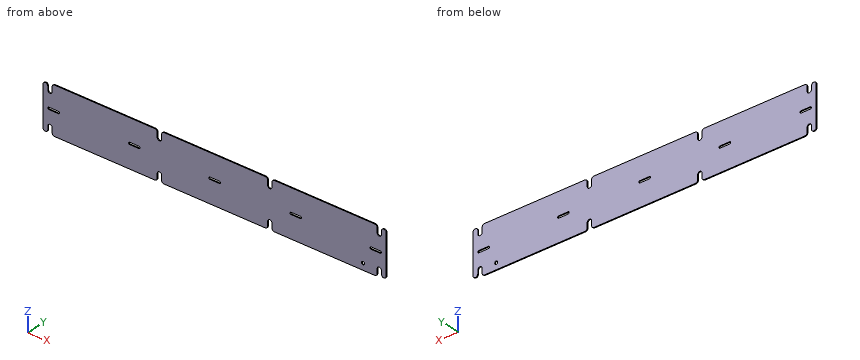
from build123d import *

# Parameters (mm, degrees)
F1_DEPTH = 1
F3_DEPTH = 25
F4_R     = 3.25
F5_DEPTH = 25


with BuildPart() as f1:
    # F0 (on Front) → F1 (new body, symmetric)
    with BuildSketch(Plane.XZ):
        with BuildLine():
            Line((-370, 42.5), (-370, -42.5))
            ThreePointArc((-370, -42.5), (-364.875, -47.501144), (-359.75, -42.5))
            Line((-359.75, -42.5), (-359.75, -35))
            ThreePointArc((-359.75, -35), (-355, -30.25), (-350.25, -35))
            Line((-350.25, -35), (-350.25, -45))
            ThreePointArc((-350.25, -45), (-348.785534, -48.535534), (-345.25, -50))
            Line((-345.25, -50), (-128.75, -50))
            ThreePointArc((-128.75, -50), (-125.214466, -48.535534), (-123.75, -45))
            Line((-123.75, -45), (-123.75, -35))
            ThreePointArc((-123.75, -35), (-119, -30.25), (-114.25, -35))
            Line((-114.25, -35), (-114.25, -45))
            ThreePointArc((-114.25, -45), (-112.785534, -48.535534), (-109.25, -50))
            Line((-109.25, -50), (109.25, -50))
            ThreePointArc((109.25, -50), (112.785534, -48.535534), (114.25, -45))
            Line((114.25, -45), (114.25, -35))
            ThreePointArc((114.25, -35), (119, -30.25), (123.75, -35))
            Line((123.75, -35), (123.75, -45))
            ThreePointArc((123.75, -45), (125.214466, -48.535534), (128.75, -50))
            Line((128.75, -50), (345.25, -50))
            ThreePointArc((345.25, -50), (348.785534, -48.535534), (350.25, -45))
            Line((350.25, -45), (350.25, -35))
            ThreePointArc((350.25, -35), (355, -30.25), (359.75, -35))
            Line((359.75, -35), (359.75, -42.5))
            ThreePointArc((359.75, -42.5), (364.875, -47.501144), (370, -42.5))
            Line((370, -42.5), (370, 42.5))
            ThreePointArc((370, 42.5), (364.875, 47.501144), (359.75, 42.5))
            Line((359.75, 42.5), (359.75, 35))
            ThreePointArc((359.75, 35), (355, 30.25), (350.25, 35))
            Line((350.25, 35), (350.25, 45))
            ThreePointArc((350.25, 45), (348.785534, 48.535534), (345.25, 50))
            Line((345.25, 50), (128.75, 50))
            ThreePointArc((128.75, 50), (125.214466, 48.535534), (123.75, 45))
            Line((123.75, 45), (123.75, 35))
            ThreePointArc((123.75, 35), (119, 30.25), (114.25, 35))
            Line((114.25, 35), (114.25, 45))
            ThreePointArc((114.25, 45), (112.785534, 48.535534), (109.25, 50))
            Line((109.25, 50), (-109.25, 50))
            ThreePointArc((-109.25, 50), (-112.785534, 48.535534), (-114.25, 45))
            Line((-114.25, 45), (-114.25, 35))
            ThreePointArc((-114.25, 35), (-119, 30.25), (-123.75, 35))
            Line((-123.75, 35), (-123.75, 45))
            ThreePointArc((-123.75, 45), (-125.214466, 48.535534), (-128.75, 50))
            Line((-128.75, 50), (-345.25, 50))
            ThreePointArc((-345.25, 50), (-348.785534, 48.535534), (-350.25, 45))
            Line((-350.25, 45), (-350.25, 35))
            ThreePointArc((-350.25, 35), (-355, 30.25), (-359.75, 35))
            Line((-359.75, 35), (-359.75, 42.5))
            ThreePointArc((-359.75, 42.5), (-364.875, 47.501144), (-370, 42.5))
        make_face()
    extrude(amount=F1_DEPTH, both=True)

    # F2 (on face) → F3 (cut)
    with BuildSketch(Plane.XZ.offset(1)):
        with BuildLine():
            Line((-357.25, -2.25), (-336.75, -2.25))
            ThreePointArc((-336.75, -2.25), (-334.5, 0), (-336.75, 2.25))
            Line((-336.75, 2.25), (-357.25, 2.25))
            ThreePointArc((-357.25, 2.25), (-359.5, 0), (-357.25, -2.25))
        make_face()
        with BuildLine():
            Line((-183.25, -2.25), (-162.75, -2.25))
            ThreePointArc((-162.75, -2.25), (-160.5, 0), (-162.75, 2.25))
            Line((-162.75, 2.25), (-183.25, 2.25))
            ThreePointArc((-183.25, 2.25), (-185.5, 0), (-183.25, -2.25))
        make_face()
        with BuildLine():
            Line((-10.25, -2.25), (10.25, -2.25))
            ThreePointArc((10.25, -2.25), (12.5, 0), (10.25, 2.25))
            Line((10.25, 2.25), (-10.25, 2.25))
            ThreePointArc((-10.25, 2.25), (-12.5, 0), (-10.25, -2.25))
        make_face()
        with BuildLine():
            Line((164.75, -2.25), (185.25, -2.25))
            ThreePointArc((185.25, -2.25), (187.5, 0), (185.25, 2.25))
            Line((185.25, 2.25), (164.75, 2.25))
            ThreePointArc((164.75, 2.25), (162.5, 0), (164.75, -2.25))
        make_face()
        with BuildLine():
            Line((336.75, -2.25), (357.25, -2.25))
            ThreePointArc((357.25, -2.25), (359.5, 0), (357.25, 2.25))
            Line((357.25, 2.25), (336.75, 2.25))
            ThreePointArc((336.75, 2.25), (334.5, 0), (336.75, -2.25))
        make_face()
    extrude(amount=-F3_DEPTH, mode=Mode.SUBTRACT)

    # F4 (on face) → F5 (cut)
    with BuildSketch(Plane.XZ.offset(1)):
        with Locations((320, -36)):
            Circle(F4_R)
    extrude(amount=-F5_DEPTH, mode=Mode.SUBTRACT)


solid = f1.part
Input: part model. Units: mm. Frame: model coordinates. Give positions to 0.01 mm unless a question says otherwise; leave off trailing zeros. Use one line per item in the form item = value.
1) First-contact query: pin 1 Ø0.6 at (x, y) = (346, 0.5) entering from +Z; pin 2 Ø10.5 at (x, z) = (320, -36) entering from +Y. Flat tips, straight axial feed; report the tip coordinate or a pass-through.
Response values:
pin_1 = 49.98
pin_2 = 1
2) Section A-A, the plane y = -0.15. Count the separate pieces of the cut face and the enclosed holes in it, and give its area (3 significant figures).
Response values:
separate_pieces = 1
enclosed_holes = 6
area = 71,800 mm^2
3) Line query: probe 1 along Z at (x, y) = (-172.5, 0.55); probe 2 along X at (y, z) = (-0.9, 39.5); probe 3 along Z at (x, y) = (320, 0.3). Output: solid intervals per line, ascending.
Response values:
probe_1 = -50 to -2.25, 2.25 to 50
probe_2 = -370 to -359.75, -350.25 to -123.75, -114.25 to 114.25, 123.75 to 350.25, 359.75 to 370
probe_3 = -50 to -39.25, -32.75 to 50
